```python
from build123d import *

# Parameters (mm, degrees)
SKETCH1_W               = 75
SKETCH1_H               = 20
BOSS_EXTRUDE1_DEPTH     = 3
SKETCH2_W               = 10
SKETCH2_H               = 100
BOSS_EXTRUDE2_DEPTH     = 10
SKETCH5_W               = 8
SKETCH5_H               = 10
SKETCH5_W_2             = 18
BOSS_EXTRUDE3_DEPTH     = 10
CUT_EXTRUDE1_DEPTH      = 117.828934772
CUT_EXTRUDE1_DEPTH_BACK = 117.828934772
SKETCH7_R               = 3.15
BOSS_EXTRUDE5_DEPTH     = 10


with BuildPart() as part:
    # Sketch1 → Boss-Extrude1 (new body)
    with BuildSketch(Plane(origin=(0, 0, 0), x_dir=(1, 0, 0), z_dir=(0, 1, 0))):
        with Locations((37.5, 10)):
            Rectangle(SKETCH1_W, SKETCH1_H)
    extrude(amount=BOSS_EXTRUDE1_DEPTH)

    # Sketch2 → Boss-Extrude2 (add)
    with BuildSketch(Plane.XY):
        with Locations((5, -50)):
            Rectangle(SKETCH2_W, SKETCH2_H)
        with Locations((70, -50)):
            Rectangle(SKETCH2_W, SKETCH2_H)
    extrude(amount=-BOSS_EXTRUDE2_DEPTH)

    # Sketch5 → Boss-Extrude3 (add)
    with BuildSketch(Plane.XY):
        with Locations((14, -95)):
            Rectangle(SKETCH5_W, SKETCH5_H)
        with Locations((56, -95)):
            Rectangle(SKETCH5_W_2, SKETCH5_H)
    extrude(amount=-BOSS_EXTRUDE3_DEPTH)

    # Sketch7 → Cut-Extrude1 (cut, two sides: drawn at the far end of the back side and taken through both)
    with BuildSketch(Plane(origin=(18, 0, 0), x_dir=(0, 0, -1), z_dir=(1, 0, 0)).offset(-CUT_EXTRUDE1_DEPTH_BACK)):
        with Locations((5, -95)):
            Circle(SKETCH7_R)
    extrude(amount=CUT_EXTRUDE1_DEPTH + CUT_EXTRUDE1_DEPTH_BACK, mode=Mode.SUBTRACT)

    # Sketch13 → Boss-Extrude5 (add)
    with BuildSketch(Plane.XY):
        Polygon((10, -24.530919021), (32.5, -24.530919021), (32.5, 0), (42.5, 0), (42.5, -24.530919021), (65, -24.530919021), (65, -34.394439552), (42.5, -34.394439552), (42.5, -45), (65, -45), (65, -55.233083722), (42.5, -55.233083722), (32.5, -55.233083722), (10, -55.233083722), (10, -45), (32.5, -45), (32.5, -34.394439552), (10, -34.394439552), align=None)
    extrude(amount=-BOSS_EXTRUDE5_DEPTH)


solid = part.part
```
Geometry: final body of the model. Coordinates: model frame, mm. A direction names the side the tool comes from. Give positions to 0.01 mm unless a question says otherwise; leave off trailing zeros. Loops run counter-clockwise (first coordinate to the right, second up) from the corner with the lowest first, then second, coordinate; pieces in that order, holes last. Notation, with made-up numbers: (18, -39) - (63, -39) arc R24 cw to (63, -22) - close; hole circle Ø8 at (29.5, 0). An arc over 180 degrees is marked (long way). Answer as CSV lines item,"result". Start each with the question number.
(1) Pin query (flat end, axial travel): P1, Ø12, axis at x = 39.5, z = -3.5, coming from the -Y side; P2, Ø3, axis at x = 61, z = -14, coming from the -Y side. Return the tip coordinate at first contact, or that it passes through.
(2) Section query D-D (y = -95). Output: boundary loops of the cut face in (x, z), and give its area (3 significant figures).
(3) Section query C-C (x = 21.5). Output: boundary loops of the cut face in (y, z), and give its area (3 significant figures).
(4) Section query B-B (y = -37.5). Output: boundary loops of the cut face in (x, z).
(5) Reachability of faces 4 (the face through (47, -98.4, -4.9)), 5 (the face through (0, -49, -5)), 6 (the face through (21, -45, -5)) from +Z, -Z, +X, -X, +Y, -Y: full face, straight path, thin tool, end or side. Return the list, or none.
(6) Ray query, line 1 along Y through (x, z) = (13.75, -5); line 2 along Y through (x, z) = (64, -9); line 3 along Z through (x, y) = (63, -95). Return the intervals inside material, ascending. Write a range as [from, to].
(7) Section query A-A (x = 49.5). Output: boundary loops of the cut face in (y, z), and give its area (3 significant figures).
(8) Mould query, pull axis Z, two halves, no side actions, for faces 1 (the face through (75, -49, -5)), 2 (the face through (8.87, -92.34, -6.69)), 3 (the face through (37, -48, 0)). Classes: +Z half, -Z half, draft (parallel to the pull), parting line (faces both ways), or undercut.
Worked answers:
1,P1,"stops at y = -55.23"
1,P2,"stops at y = 0"
2,outline,"(0, -10) - (18, -10) - (18, -8.15) - (0, -8.15) - close; (0, -1.85) - (18, -1.85) - (18, 0) - (0, 0) - close; (47, -10) - (75, -10) - (75, -8.15) - (47, -8.15) - close; (47, -1.85) - (75, -1.85) - (75, 0) - (47, 0) - close"
2,area,"170 mm^2"
3,outline,"(-55.23, -10) - (-45, -10) - (-45, 0) - (-55.23, 0) - close; (-34.39, -10) - (-24.53, -10) - (-24.53, 0) - (-34.39, 0) - close; (0, -20) - (3, -20) - (3, 0) - (0, 0) - close"
3,area,"261 mm^2"
4,outline,"(0, -10) - (10, -10) - (10, 0) - (0, 0) - close; (32.5, -10) - (42.5, -10) - (42.5, 0) - (32.5, 0) - close; (65, -10) - (75, -10) - (75, 0) - (65, 0) - close"
5,face 4,"+Z, -Z, -Y"
5,face 5,"+Z, -Z, -X, +Y, -Y"
5,face 6,"+Z, -Z"
6,line 1,"y = [-100, -98.15], [-91.85, -90], [-55.23, -45], [-34.39, -24.53], [0, 3]"
6,line 2,"y = [-100, -90], [-55.23, -45], [-34.39, -24.53], [0, 3]"
6,line 3,"z = [-10, -8.15], [-1.85, 0]"
7,outline,"(-100, -10) - (-90, -10) - (-90, 0) - (-100, 0) - close; (-55.23, -10) - (-45, -10) - (-45, 0) - (-55.23, 0) - close; (-34.39, -10) - (-24.53, -10) - (-24.53, 0) - (-34.39, 0) - close; (0, -20) - (3, -20) - (3, 0) - (0, 0) - close; hole circle Ø6.3 at (-95, -5)"
7,area,"330 mm^2"
8,face 1,"draft"
8,face 2,"undercut"
8,face 3,"+Z half"
